Part model, mm, in its own coordinate system. A direction names the side the tool comes from. Round coordinates to 2 decimals unless told otherwise and drop trailing zeros. Loops run counter-clockwise (first coordinate to the right, second up) from the corner with the lowest first, then second, coordinate; pieces in that order, holes last.
1) Band-saw the part on B-B, the plane x = 88. Write the cut outline in (y, z) (3 decimals).
2) Mould opens along X. For faces 4 (the flat face through (89.887, 23, 52)), 5 (the flat face through (66, 0, 42.875)), 6 (the flat face through (22.225, 0, 18)) say: +X half, -X half, draft (parallel to the pull), parting line (faces both ways), or undercut.
3) Band-saw the part on A-A, the plane y = 0. Write the cut outline in (x, z) (3 decimals).
4) Band-saw the part on C-C, the plane z = 34.5. Write the cut outline in (x, y), then the cut area to 3 significant figures.
5) Drop flat-ended pins along their axis: P1, Ø2, axis at y = -22.5, z = 56, coming from the +X side; P2, Ø1.5, axis at y = -19, z = 51.5, coming from the +X side; P3, Ø2, axis at y = -7, z = 49, coming from the +X side. Give the stop position or say it passes through.
6) Band-saw the part on D-D, the plane y = 31. Write the cut outline in (x, z) (3 decimals).
7) Probe line 1 (X direction, y = 21.5, z = 14) (3 decimals); line 2 (Z direction, x = -16.5, y = -36.5) (3 decimals); line 3 (X direction, y = 51, z = -2.5) (3 decimals). List the from-to ranges inside material, lowest first.
8) 3-axis set-ups, long thin cutter, end or side, ignore diameter. For faces 1 (the cylindrical face through (45.8, -0.4, 38.1)), 2 (the flat face through (90, 0, 38.1)), 3 (the flat face through (48, 25.4, 42)): which of +Z, -Z, +X, -X, +Y, -Y reach the whole face in a straight line?
from build123d import *

# Parameters (mm, degrees)
F1_DEPTH = 63.5
F0_W     = 29.5617593795
F0_H     = 19.05
F2_DEPTH = 25.4
F5_R     = 6.35


# Not quite as in the source:
# - a feature of the source that left no trace in its solid (it failed there, or was rolled back) is left out


with BuildPart() as f1:
    # F0 (on Front) → F1 (new body, symmetric)
    with BuildSketch(Plane.XZ):
        Polygon((41.275, -9.525), (41.275, 9.525), (22.225, 9.525), (-41.275, 9.525), (-41.275, -9.525), align=None)
    extrude(amount=F1_DEPTH, both=True)

    # F0 (on Front) → F2 (join, symmetric)
    with BuildSketch(Plane.XZ):
        with BuildLine():
            Line((22.225, 9.525), (41.275, 9.525))
            Line((41.275, 9.525), (41.275, 27.0002))
            ThreePointArc((41.275, 27.0002), (45.9246798487, 38.2255201513), (57.15, 42.8752))
            Line((57.15, 42.8752), (60.325, 42.8752))
            Line((60.325, 42.8752), (60.325, 61.9252))
            Line((60.325, 61.9252), (57.15, 61.9252))
            ThreePointArc((57.15, 61.9252), (32.4542956671, 51.6959043329), (22.225, 27.0002))
            Line((22.225, 27.0002), (22.225, 9.525))
        make_face()
        with Locations((75.1058796897, 52.4002)):
            Rectangle(F0_W, F0_H)
    extrude(amount=F2_DEPTH, both=True)

    # F0 (on Front) → F4 (revolve)
    with BuildSketch(Plane.XZ):
        Polygon((89.8867593795, 61.9252), (89.8867593795, 42.8752), (89.8867593795, 38.1), (111.125, 38.1), (111.125, 66.675), (89.8867593795, 66.675), align=None)
    revolve(axis=Axis((89.8867593795, 0, 52.3875), (0, 0, 1)))

    # F5
    f5_edges = [f1.edges().sort_by_distance(p)[0] for p in [
        (41.275, -63.5, 0),
        (-41.275, -63.5, 0),
        (41.275, 63.5, 0),
        (-41.275, 63.5, 0),
    ]]
    fillet(f5_edges, radius=F5_R)


solid = f1.part
Reported:
1. outline: (-25.4, 42.875) - (-21.154, 42.875) - (-21.154, 38.1) - (21.154, 38.1) - (21.154, 42.875) - (25.4, 42.875) - (25.4, 61.925) - (21.154, 61.925) - (21.154, 66.675) - (-21.154, 66.675) - (-21.154, 61.925) - (-25.4, 61.925) - close
2. face 4: +X half
2. face 5: undercut
2. face 6: -X half
3. outline: (-41.275, -9.525) - (41.275, -9.525) - (41.275, 27) arc R15.875 cw to (57.15, 42.875) - (68.649, 42.875) - (68.649, 38.1) - (111.125, 38.1) - (111.125, 66.675) - (68.649, 66.675) - (68.649, 61.925) - (57.15, 61.925) arc R34.925 ccw to (22.225, 27) - (22.225, 9.525) - (-41.275, 9.525) - close
4. outline: (23.04, -25.4) - (43.16, -25.4) - (43.16, 25.4) - (23.04, 25.4) - close
4. area: 1,020 mm2
5. P1: stops at x = 89.89
5. P2: stops at x = 100.75
5. P3: stops at x = 110.26
6. outline: (-41.275, -9.525) - (41.275, -9.525) - (41.275, 9.525) - (-41.275, 9.525) - close
7. line 1: x = 22.225 to 41.275
7. line 2: z = -9.525 to 9.525
7. line 3: x = -41.275 to 41.275
8. face 1: -Z, +Y, -Y
8. face 2: -Z, +X, +Y, -Y
8. face 3: +Z, +X, -X, +Y
